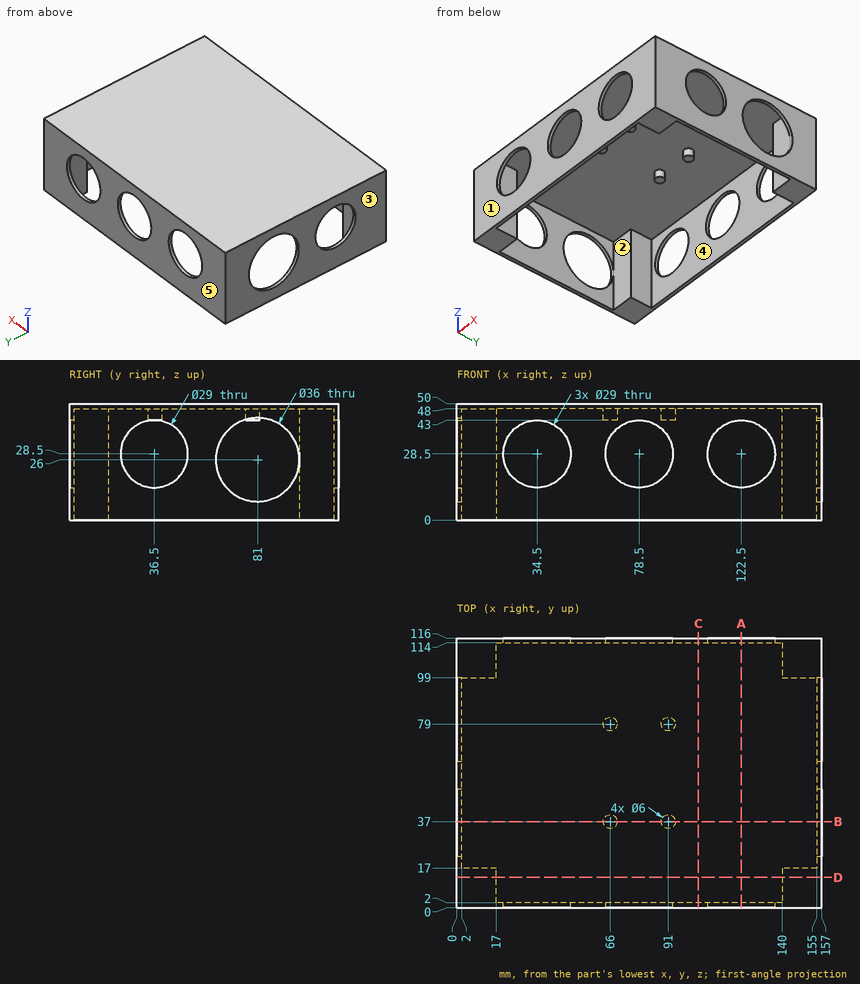
Geometry: see drawing. Coordinates: mm, zero at the bounding-box minimum. A direction names the side the tool comes from. Coordinates: 2 decimals unless noted, no trailing zeros. Loops run counter-clockwise (first coordinate to the right, second up) from the corner with the lowest first, then second, coordinate; pieces in that order, holes last. Notation, with made-up numbers: M 86.25,11 L 143.25,11 A12 cw 143.25,23 Z; hole C 28,-32 d8. An arc over 180 degrees is marked long. Answer in a Markdown table with one row per item.
Q1. Section B-B on y = 37. Return the cut outline in (x, z), plus the area to 3 significant figures.
Answers below:
| item | result |
|---|---|
| outline | M 0,0 L 2,0 L 2,14.01 L 0,14.01 Z; M 0,42.99 L 2,42.99 L 2,48 L 63,48 L 63,43 L 69,43 L 69,48 L 88,48 L 88,43 L 94,43 L 94,48 L 155,48 L 155,42.99 L 157,42.99 L 157,50 L 0,50 Z; M 155,0 L 157,0 L 157,14.01 L 155,14.01 Z |
| area | 450 mm^2 |
Q2. Section C-C on x = 104. Return the cut outline in (y, z), plus the area to 3 significant figures.
Answers below:
| item | result |
|---|---|
| outline | M 0,0 L 2,0 L 2,48 L 114,48 L 114,0 L 116,0 L 116,50 L 0,50 Z |
| area | 424 mm^2 |
Q3. Ray query, probe 1 along X at (y, z) = (114.55, 28.5); probe 2 along Y at (x, z) = (101, 19.5); probe 3 along X at (y, z) = (59, 6). Return the intervals inside material, ascending. Write a range as from..to.
Answers below:
| item | result |
|---|---|
| probe 1 | x = 0..20, 49..64, 93..108, 137..157 |
| probe 2 | y = 0..2, 114..116 |
| probe 3 | x = 0..2, 155..157 |
Q4. Section D-D on y = 13. Return the cut outline in (x, z).
Answers below:
| item | result |
|---|---|
| outline | M 0,0 L 17,0 L 17,48 L 140,48 L 140,0 L 157,0 L 157,50 L 0,50 Z |
Q5. Draft query along Y for the marked faces 1, 2 and 3. Return one class per face: pulls with the +Y half, pulls with the -Y half, needs draft (parallel to the pull), parting line crosses it, or undercut.
Answers below:
| item | result |
|---|---|
| face 1 | pulls with the -Y half |
| face 2 | undercut |
| face 3 | needs draft |
Q6. First-contact query: pin 1 (1.5 mm diameter, centred on x = 26, y = 38, fed in from -Z); pin 2 (5 mm diameter, centred on x = 92, y = 79, fed in from -Z). Flat tips, straight axial feed; report the tip coordinate or a pass-through.
Answers below:
| item | result |
|---|---|
| pin 1 | stops at z = 48 |
| pin 2 | stops at z = 43 |
Q7. Set-up query: the marked faces 4 and 5. Return all of +Z, -Z, +X, -X, +Y, -Y with unobstructed straight access to the full face (end or side cutting, diameter ignored); none if empty.
Answers below:
| item | result |
|---|---|
| face 4 | -Z |
| face 5 | +Z, -Z, +X, -X, +Y |
Q8. Section A-A on x = 122.5. Return the cut outline in (y, z).
Answers below:
| item | result |
|---|---|
| outline | M 0,0 L 2,0 L 2,14 L 0,14 Z; M 0,43 L 2,43 L 2,48 L 114,48 L 114,43 L 116,43 L 116,50 L 0,50 Z; M 114,0 L 116,0 L 116,14 L 114,14 Z |
